```python
from build123d import *

# Parameters (mm, degrees)
F1_DEPTH     = 10
F2_R         = 2
F3_T1_DEPTH  = 15
F3_T3_DEPTH  = 6
F3_T5_DEPTH  = 36
F3_S9_W      = 2
F3_S9_H      = 2
F3_T10_DEPTH = 2
F3_S15_W     = 2
F3_S15_H     = 2
F3_T16_DEPTH = 2
F3_S21_W     = 2
F3_S21_H     = 2
F3_T22_DEPTH = 2
F3_S27_W     = 2
F3_S27_H     = 2
F3_T28_DEPTH = 2


# Not quite as in the source:
# - a fillet or chamfer that OpenCascade refuses, or shapes differently, is made with other operations: its cross-section is extruded or revolved along the edge and cut away or added


with BuildPart() as f1:
    # F0 (on Top) → F1 (new body)
    with BuildSketch(Plane.XY):
        with BuildLine():
            Line((40, 17.25), (0, 17.25))
            Line((0, 17.25), (0, 5.25))
            Line((0, 5.25), (19, 5.25))
            ThreePointArc((19, 5.25), (20, 6.25), (21, 5.25))
            Line((21, 5.25), (40, 5.25))
            Line((40, 5.25), (40, 17.25))
        make_face()
    extrude(amount=F1_DEPTH)

    # F2
    f2_edges = [f1.edges().sort_by_distance(p)[0] for p in [
        (0, 11.25, 0),
        (0, 11.25, 10),
        (0, 17.25, 5),
    ]]
    fillet(f2_edges, radius=F2_R)

    # F3: fillet of radius 2 on 5 edges, made by hand

    # F3_s2 → F3_t1 (cut)
    with BuildSketch(Plane.XZ.offset(-15.25)):
        with BuildLine():
            ThreePointArc((38, 0), (39.4142135624, 0.5857864376), (40, 2))
            Line((40, 2), (40, 0))
            Line((40, 0), (38, 0))
        make_face()
        with BuildLine():
            ThreePointArc((40, 8), (39.4142135624, 9.4142135624), (38, 10))
            Line((38, 10), (40, 10))
            Line((40, 10), (40, 8))
        make_face()
    extrude(amount=F3_T1_DEPTH, mode=Mode.SUBTRACT)

    # F3_s4 → F3_t3 (cut)
    with BuildSketch(Plane.XY.offset(2)):
        with BuildLine():
            ThreePointArc((38, 17.25), (39.4142135624, 16.6642135624), (40, 15.25))
            Line((40, 15.25), (40, 17.25))
            Line((40, 17.25), (38, 17.25))
        make_face()
    extrude(amount=F3_T3_DEPTH, mode=Mode.SUBTRACT)

    # F3_s6 → F3_t5 (cut)
    with BuildSketch(Plane.YZ.offset(2)):
        with BuildLine():
            ThreePointArc((17.25, 2), (16.6642135624, 0.5857864376), (15.25, 0))
            Line((15.25, 0), (17.25, 0))
            Line((17.25, 0), (17.25, 2))
        make_face()
        with BuildLine():
            ThreePointArc((17.25, 8), (16.6642135624, 9.4142135624), (15.25, 10))
            Line((15.25, 10), (17.25, 10))
            Line((17.25, 10), (17.25, 8))
        make_face()
    extrude(amount=F3_T5_DEPTH, mode=Mode.SUBTRACT)


with BuildPart() as f3_tool8:
    # F3_s9 → F3_t10 (new body)
    with BuildSketch(Plane.XZ.offset(-15.25)):
        with Locations((1, 9)):
            Rectangle(F3_S9_W, F3_S9_H)
    extrude(amount=-F3_T10_DEPTH)

    # F3_s11 → F3_t12 (revolve, cut)
    with BuildSketch(Plane(origin=(2, 15.25, 8), x_dir=(0.7071067812, 0, -0.7071067812), z_dir=(0.7071067812, 0, 0.7071067812))):
        with BuildLine():
            ThreePointArc((0, -2), (2, 0), (0, 2))
            Line((0, 2), (0, -2))
        make_face()
    revolve(axis=Axis((2, 15.25, 8), (0, 1, 0)), mode=Mode.SUBTRACT)


with BuildPart() as f1_1:
    add(f1.part)

    # F3_t7: cut F3_tool8
    add(f3_tool8.part, mode=Mode.SUBTRACT)


with BuildPart() as f3_tool14:
    # F3_s15 → F3_t16 (new body)
    with BuildSketch(Plane.XZ.offset(-15.25)):
        with Locations((1, 1)):
            Rectangle(F3_S15_W, F3_S15_H)
    extrude(amount=-F3_T16_DEPTH)

    # F3_s17 → F3_t18 (revolve, cut)
    with BuildSketch(Plane(origin=(2, 15.25, 2), x_dir=(0.7071067812, 0, 0.7071067812), z_dir=(-0.7071067812, 0, 0.7071067812))):
        with BuildLine():
            ThreePointArc((0, -2), (2, 0), (0, 2))
            Line((0, 2), (0, -2))
        make_face()
    revolve(axis=Axis((2, 15.25, 2), (0, 1, 0)), mode=Mode.SUBTRACT)


with BuildPart() as f1_2:
    add(f1_1.part)

    # F3_t13: cut F3_tool14
    add(f3_tool14.part, mode=Mode.SUBTRACT)


with BuildPart() as f3_tool20:
    # F3_s21 → F3_t22 (new body)
    with BuildSketch(Plane.XZ.offset(-15.25)):
        with Locations((39, 1)):
            Rectangle(F3_S21_W, F3_S21_H)
    extrude(amount=-F3_T22_DEPTH)

    # F3_s23 → F3_t24 (revolve, cut)
    with BuildSketch(Plane(origin=(38, 15.25, 2), x_dir=(-0.7071067812, 0, 0.7071067812), z_dir=(-0.7071067812, 0, -0.7071067812))):
        with BuildLine():
            ThreePointArc((0, -2), (2, 0), (0, 2))
            Line((0, 2), (0, -2))
        make_face()
    revolve(axis=Axis((38, 15.25, 2), (0, 1, 0)), mode=Mode.SUBTRACT)


with BuildPart() as f1_3:
    add(f1_2.part)

    # F3_t19: cut F3_tool20
    add(f3_tool20.part, mode=Mode.SUBTRACT)


with BuildPart() as f3_tool26:
    # F3_s27 → F3_t28 (new body)
    with BuildSketch(Plane.XZ.offset(-15.25)):
        with Locations((39, 9)):
            Rectangle(F3_S27_W, F3_S27_H)
    extrude(amount=-F3_T28_DEPTH)

    # F3_s29 → F3_t30 (revolve, cut)
    with BuildSketch(Plane(origin=(38, 15.25, 8), x_dir=(-0.7071067812, 0, -0.7071067812), z_dir=(0.7071067812, 0, -0.7071067812))):
        with BuildLine():
            ThreePointArc((0, -2), (2, 0), (0, 2))
            Line((0, 2), (0, -2))
        make_face()
    revolve(axis=Axis((38, 15.25, 8), (0, 1, 0)), mode=Mode.SUBTRACT)


with BuildPart() as f1_4:
    add(f1_3.part)

    # F3_t25: cut F3_tool26
    add(f3_tool26.part, mode=Mode.SUBTRACT)


solid = f1_4.part
```
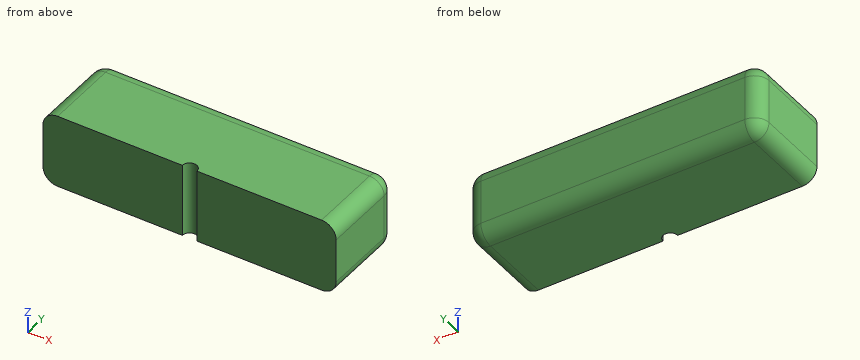
Check sheet for the modelled part. Datum: model origin and axes. Units: mm. Round coordinates to 2 decimals unless told otherwise and drop trailing zeros. Loops run counter-clockwise (first coordinate to the right, second up) from the corner with the lowest first, then second, coordinate; pieces in that order, holes last. Notation, with made-up numbers: (-11.75, 84) - (26.25, 84) arc R22 cw to (26.25, 97) - close; hole circle Ø2 at (87, 62). An arc over 180 degrees is marked (long way). Answer as a JSON object with one key per item and string values. Group by question number.
Q1. Gauge pin test, flat end, axial feed: P1, Ø1, axis at x = 4.5, y = 16, coming from the -Z side. Record the tip position at first contact, or that the pin passes through.
Q2. Scan lines: line 1 along X through (y, z) = (6, 6); line 2 along Y through (x, z) = (15, 8.5); line 3 along X through (y, z) = (7.5, 9). Record each from-to range of solid material in increasing order. Write a range as [from, to].
Q3. Sectioned sample at A-A, the plane x = 20. Enter the section's corners in (y, z), plus the area to 3 significant figures.
Solution:
{
 "1": {"P1": "stops at z = 0.02"},
 "2": {"line 1": "x = [0, 19.34], [20.66, 40]", "line 2": "y = [5.25, 17.19]", "line 3": "x = [0.27, 39.73]"},
 "3": {"outline": "(6.25, 0) - (15.25, 0) arc R2 ccw to (17.25, 2) - (17.25, 8) arc R2 ccw to (15.25, 10) - (6.25, 10) - close", "area": "108 mm²"}
}
